Source: three-view drawing plus pictorial views. Frame: mm from the lowest corner of the part. Give positions to 0.01 mm unless a question says otherwise; leave off trailing zeros. Loops run counter-clockwise (first coordinate to the right, second up) from the corner with the lowest first, then second, coordinate; pieces in that order, holes last. Notation, with made-up numbers: M 28.5,54.25 L 60.5,54.25 A21 ccw 60.5,70.25 Z; hole C -16.5,64 d8. An arc over 180 degrees is marked long. Put each result on its own line as item: value. Start each with the question number.
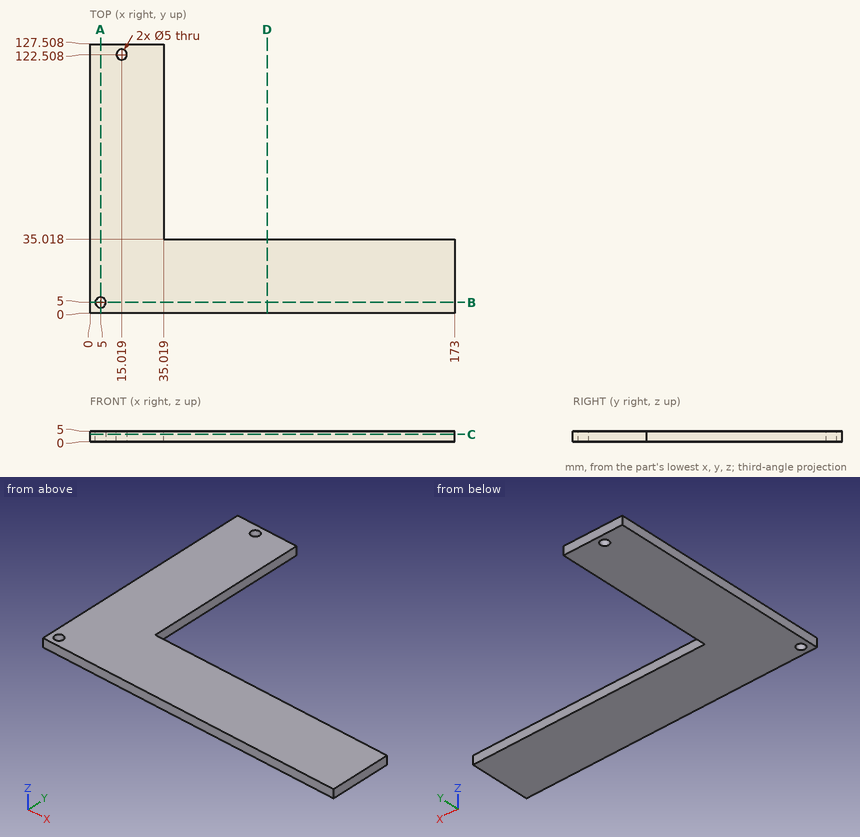
1. Ray query, line 1 (Y direction, x = 5, z = 2.1); line 2 (Y direction, x = 88.5, z = 3.8); line 3 (Y direction, x = 7, z = 2.55). Return the intervals inside material, ascending.
2. Contact query for a flat-ended pin moving along its axis: pin 1 (1.5 mm diameter, centred on x = 102.5, z = 1.5, fed in from +Y). Output: stop coordinate, or through.
3. Section B-B, the plane y = 5. Output: boundary loops of the cut face in (x, z), plus the area to 3 significant figures.
4. Section A-A, the plane x = 5. Output: boundary loops of the cut face in (y, z).
5. Section D-D, the plane x = 84. Output: boundary loops of the cut face in (y, z).
6. Section C-C, the plane z = 3.4. Output: boundary loops of the cut face in (x, y), plus the area to 3 significant figures.
Results found:
1. line 1: 0 to 2.5, 7.5 to 127.51
1. line 2: 0 to 35.02
1. line 3: 0 to 3.5, 6.5 to 127.51
2. pin 1: y = 35.02
3. outline: M 0,0 L 2.5,0 L 2.5,5 L 0,5 Z; M 7.5,0 L 173,0 L 173,5 L 7.5,5 Z
3. area: 840 mm²
4. outline: M 0,0 L 2.5,0 L 2.5,5 L 0,5 Z; M 7.5,0 L 127.51,0 L 127.51,5 L 7.5,5 Z
5. outline: M 0,0 L 35.02,0 L 35.02,5 L 0,5 Z
6. outline: M 0,0 L 173,0 L 173,35.02 L 35.02,35.02 L 35.02,127.51 L 0,127.51 Z; hole C 5,5 d5; hole C 15.02,122.51 d5
6. area: 9,260 mm²
